from build123d import *

# Parameters (mm, degrees)
SKETCH1_W               = 2
SKETCH1_H               = 20.42
BOSS_EXTRUDE1_DEPTH     = 4.62
BOSS_EXTRUDE1_2_DEPTH   = 4.62
SKETCH2_W               = 16.1
SKETCH2_H               = 1.1
BOSS_EXTRUDE2_DEPTH     = 8.57
SKETCH3_W               = 20.1
SKETCH3_H               = 1.5
BOSS_EXTRUDE3_DEPTH     = 4.62
SKETCH4_W               = 16.1
SKETCH4_H               = 1.5
BOSS_EXTRUDE4_DEPTH     = 3.95
SKETCH5_W               = 19.32
SKETCH5_H               = 1.5
BOSS_EXTRUDE5_DEPTH     = 16.1
SKETCH6_W               = 11.5
SKETCH6_H               = 11.5
CUT_EXTRUDE1_DEPTH      = 18.651388047
SKETCH8_W               = 2.2
SKETCH8_H               = 0.55
CUT_EXTRUDE2_DEPTH      = 3.95
SKETCH10_W              = 8.121119636
SKETCH10_H              = 3.071119636
CUT_EXTRUDE3_DEPTH      = 1.5
SKETCH11_W              = 16.1
SKETCH11_H              = 2.3
BOSS_EXTRUDE6_DEPTH     = 2.08
CUT_EXTRUDE5_START      = -7.07
SKETCH12_W              = 16.1
SKETCH12_H              = 0.4
CUT_EXTRUDE5_DEPTH      = 7.07
CUT_EXTRUDE6_DEPTH      = 24.21892547
CUT_EXTRUDE6_DEPTH_BACK = 24.21892547
SKETCH13_W              = 0.2
SKETCH13_H              = 2.3
SKETCH14_W              = 0.474033505
SKETCH14_H              = 2.3
CUT_EXTRUDE8_DEPTH      = 24.100703452


with BuildPart() as part:
    # Sketch1 → Boss-Extrude1 (new body)
    with BuildSketch(Plane(origin=(0, 0, 0), x_dir=(1, 0, 0), z_dir=(0, 1, 0))):
        with Locations((-9.05, 0)):
            Rectangle(SKETCH1_W, SKETCH1_H)
    extrude(amount=BOSS_EXTRUDE1_DEPTH)



with BuildPart() as body_2:
    # Sketch1 → Boss-Extrude1 2 (new body)
    with BuildSketch(Plane(origin=(0, 0, 0), x_dir=(1, 0, 0), z_dir=(0, 1, 0))):
        with Locations((9.05, 0)):
            Rectangle(SKETCH1_W, SKETCH1_H)
    extrude(amount=BOSS_EXTRUDE1_2_DEPTH)


with BuildPart() as part_1:
    add(part.part)

    add(body_2.part)  # Boss-Extrude2 merges body 2
    # Sketch2 → Boss-Extrude2 (add)
    with BuildSketch(Plane(origin=(0, 4.62, 0), x_dir=(1, 0, 0), z_dir=(0, 1, 0))):
        with Locations((0, -9.66)):
            Rectangle(SKETCH2_W, SKETCH2_H)
    extrude(amount=-BOSS_EXTRUDE2_DEPTH)

    # Sketch3 → Boss-Extrude3 (add)
    with BuildSketch(Plane(origin=(0, 4.62, 0), x_dir=(1, 0, 0), z_dir=(0, 1, 0))):
        with Locations((0, 10.96)):
            Rectangle(SKETCH3_W, SKETCH3_H)
    extrude(amount=-BOSS_EXTRUDE3_DEPTH)

    # Sketch4 → Boss-Extrude4 (add)
    with BuildSketch(Plane.XZ):
        with Locations((0, -10.96)):
            Rectangle(SKETCH4_W, SKETCH4_H)
    extrude(amount=BOSS_EXTRUDE4_DEPTH)

    # Sketch5 → Boss-Extrude5 (add)
    with BuildSketch(Plane(origin=(-8.05, 0, 0), x_dir=(0, 0, -1), z_dir=(1, 0, 0))):
        with Locations((0.55, 3.87)):
            Rectangle(SKETCH5_W, SKETCH5_H)
    extrude(amount=BOSS_EXTRUDE5_DEPTH)

    # Sketch6 → Cut-Extrude1 (cut, through all)
    with BuildSketch(Plane(origin=(0, 4.62, 0), x_dir=(1, 0, 0), z_dir=(0, 1, 0))):
        with Locations((0, -1.86)):
            Rectangle(SKETCH6_W, SKETCH6_H)
    extrude(amount=-CUT_EXTRUDE1_DEPTH, mode=Mode.SUBTRACT)

    # Sketch8 → Cut-Extrude2 (cut)
    with BuildSketch(Plane(origin=(0, 4.62, 0), x_dir=(1, 0, 0), z_dir=(0, 1, 0))):
        with Locations((0, -7.885)):
            Rectangle(SKETCH8_W, SKETCH8_H)
        with Locations((-2.55, 4.165)):
            Rectangle(SKETCH8_W, SKETCH8_H)
        with Locations((2.55, 4.165)):
            Rectangle(SKETCH8_W, SKETCH8_H)
    extrude(amount=-CUT_EXTRUDE2_DEPTH, mode=Mode.SUBTRACT)

    # Sketch10 → Cut-Extrude3 (cut)
    with BuildSketch(Plane(origin=(0, 0, -11.71), x_dir=(-1, 0, 0), z_dir=(0, 0, -1))):
        with Locations((0.420559818, 0.564440182)):
            Rectangle(SKETCH10_W, SKETCH10_H)
    extrude(amount=-CUT_EXTRUDE3_DEPTH, mode=Mode.SUBTRACT)

    # Sketch11 → Boss-Extrude6 (add)
    with BuildSketch(Plane(origin=(0, 0, -11.71), x_dir=(-1, 0, 0), z_dir=(0, 0, -1))):
        with Locations((0, -2.8)):
            Rectangle(SKETCH11_W, SKETCH11_H)
    extrude(amount=BOSS_EXTRUDE6_DEPTH)

    # Sketch12 → Cut-Extrude5 (cut)
    with BuildSketch(Plane.XZ.offset(3.95).offset(CUT_EXTRUDE5_START)):
        with Locations((0, -10.41)):
            Rectangle(SKETCH12_W, SKETCH12_H)
    extrude(amount=CUT_EXTRUDE5_DEPTH, mode=Mode.SUBTRACT)

    # Sketch13 → Cut-Extrude6 (cut, two sides: drawn at the far end of the back side and taken through both)
    with BuildSketch(Plane.ZY.offset(8.05).offset(-CUT_EXTRUDE6_DEPTH_BACK)):
        with Locations((-13.69, -2.8)):
            Rectangle(SKETCH13_W, SKETCH13_H)
    extrude(amount=CUT_EXTRUDE6_DEPTH + CUT_EXTRUDE6_DEPTH_BACK, mode=Mode.SUBTRACT)

    # Sketch14 → Cut-Extrude8 (cut, through all)
    with BuildSketch(Plane.ZY.offset(8.05)):
        with Locations((-13.352983248, -2.8)):
            Rectangle(SKETCH14_W, SKETCH14_H)
    extrude(amount=-CUT_EXTRUDE8_DEPTH, mode=Mode.SUBTRACT)


solid = part_1.part
Input: part model. Units: mm. Frame: model coordinates. A direction names the side the tool comes from. Coordinates: 2 decimals unless noted, no trailing zeros. Write each loop counter-clockwise with the first axis right and the second up, starting at its lowest first coordinate (ties: lowest second). Pieces come first, ordered by that corner, then holes. Notation, with made-up numbers: M -28.5,38.5 L -1.5,38.5 A38 ccw -1.5,76.5 Z; hole C -14,74 d9. An arc over 180 degrees is marked long. Answer as a JSON object with one key per item and string values. Group by question number.
(1) Mould query, pull axis Z, two halves, no side actions, for faces 5 (the face through (-3, 4, 7.61)), 6 (the face through (0, 3, -11.71)), 7 (the face through (3.64, 1, -11)), 8 (the face through (0, 0, 10.21)). Classes: pulls with the +Z half, pulls with the -Z half, needs draft (parallel to the pull), parting line crosses it, or undercut.
(2) Contact query for flat-ended pins moving along their axis: P1, Ø4, axis at y = -1, z = -8, coming from the -X side; P2, Ø1.3, axis at y = -1.5, z = -12.5, coming from the -X side; P3, Ø2, axis at x = 9.5, z = -4, coming from the -Y side; P4, Ø1.2, axis at y = -3, z = 9.5, coming from the +X side. Output: stop coordinate, or through.
(3) Section C-C on z = -3. Output: boundary loops of the cut face in (x, y), plus the area to 3 significant figures.
(4) Section B-B on x = 2.25. Output: boundary loops of the cut face in (y, z).
(5) Ray query, line 1 along X through (y, z) = (3.25, -0.5); line 2 along Z through (x, y) = (4.25, -2.75); line 3 along Z through (x, y) = (-3.75, 3). Return the intervals inside material, ascending. Write a range as [from, to].
(6) Set-up query: faces 1 (the face through (0, -1.65, -12)), 2 (the face through (0, -0.971, -11)), 3 (the face through (-5, 4, -3.89)), 4 (the face through (-8.05, 2, -1)). Return all of +Z, -Z, +X, -X, +Y, -Y with unobstructed straight access to the full face (end or side cutting, diameter ignored); none if empty.
(7) Section A-A on x = -5. Output: boundary loops of the cut face in (y, z), plus the area to 3 significant figures.
(8) Section D-D on y = -0.5. Output: boundary loops of the cut face in (x, z), plus the area to 3 significant figures.
Result set:
{
 "1": {"face 5": "undercut", "face 6": "pulls with the -Z half", "face 7": "needs draft", "face 8": "pulls with the +Z half"},
 "2": {"P1": "stops at x = -10.05", "P2": "stops at x = -8.05", "P3": "stops at y = 0", "P4": "stops at x = 8.05"},
 "3": {"outline": "M -10.05,0 L -8.05,0 L -8.05,3.12 L -5.75,3.12 L -5.75,4.62 L -10.05,4.62 Z; M 5.75,3.12 L 8.05,3.12 L 8.05,0 L 10.05,0 L 10.05,4.62 L 5.75,4.62 Z", "area": "25.4 mm2"},
 "4": {"outline": "M -3.95,-13.12 L -1.65,-13.12 L -1.65,-11.71 L -0.97,-11.71 L -0.97,-10.61 L -3.95,-10.61 Z; M -3.95,9.11 L 3.12,9.11 L 3.12,7.61 L 4.62,7.61 L 4.62,10.21 L -3.95,10.21 Z; M 2.1,-11.71 L 4.62,-11.71 L 4.62,-4.44 L 3.12,-4.44 L 3.12,-10.61 L 2.1,-10.61 Z"},
 "5": {"line 1": "x = [-10.05, -5.75], [5.75, 10.05]", "line 2": "z = [-13.12, -10.61], [9.11, 10.21]", "line 3": "z = [-11.71, -10.61], [9.11, 10.21]"},
 "6": {"face 1": "-Z, +X, -X, +Y", "face 2": "-Z", "face 3": "+Y, -Y", "face 4": "-Y"},
 "7": {"outline": "M -3.95,-13.12 L -1.65,-13.12 L -1.65,-11.71 L 4.62,-11.71 L 4.62,-3.89 L 3.12,-3.89 L 3.12,-10.61 L -3.95,-10.61 Z; M -3.95,9.11 L 3.12,9.11 L 3.12,7.61 L 4.62,7.61 L 4.62,10.21 L -3.95,10.21 Z", "area": "34.4 mm2"},
 "8": {"outline": "M -8.05,-11.71 L -4.48,-11.71 L -4.48,-10.61 L -8.05,-10.61 Z; M -8.05,9.11 L 8.05,9.11 L 8.05,10.21 L -8.05,10.21 Z; M 3.64,-11.71 L 8.05,-11.71 L 8.05,-10.61 L 3.64,-10.61 Z", "area": "26.5 mm2"}
}
